Can you work these out from the model? Positions are in its coordinate system, mm. A direction names the side the tool comes from. Coordinates: 2 decimals unless noted, no trailing zeros. Order: outer loops, then holes, each group sorted by start corner. A loop starts at its lowest first (then second) coordinate and runs counter-clockwise, first axis right, second up.
```python
from build123d import *

# Parameters (mm, degrees)
SKETCH1_R      = 2.15
EXTRUDE1_DEPTH = 3


with BuildPart() as part:
    # Sketch1 → Extrude1 (new body)
    with BuildSketch(Plane.XY):
        Polygon((52.497048214, 165), (-27.502951786, 165), (-27.502951786, 115), (-7.502951786, 115), (-7.502951786, 125), (12.497048214, 145), (52.497048214, 145), align=None)
        with Locations((2.497048214, 155)):
            Circle(SKETCH1_R, mode=Mode.SUBTRACT)
        with Locations((42.497048214, 155)):
            Circle(SKETCH1_R, mode=Mode.SUBTRACT)
        with Locations((-17.502951786, 125)):
            Circle(SKETCH1_R, mode=Mode.SUBTRACT)
        with Locations((-17.502951786, 155)):
            Circle(SKETCH1_R, mode=Mode.SUBTRACT)
    extrude(amount=EXTRUDE1_DEPTH)


solid = part.part
```
1. Imagine slicing it at D-D on x = -3.5. Please give me the cut outline in (y, z), then the cut area to 3 significant figures.
Completed:
outline: (129, 0) - (165, 0) - (165, 3) - (129, 3) - close
area: 108 mm2
2. Imagine slicing it at B-B on z = 1.6. Please give me the cut outline in (x, y).
Completed:
outline: (-27.5, 115) - (-7.5, 115) - (-7.5, 125) - (12.5, 145) - (52.5, 145) - (52.5, 165) - (-27.5, 165) - close; hole circle Ø4.3 at (-17.5, 125); hole circle Ø4.3 at (-17.5, 155); hole circle Ø4.3 at (2.5, 155); hole circle Ø4.3 at (42.5, 155)
3. Thinking about a two-plate mould opening in Y: for faces 3 (the cylindrical face through (43.5, 153.1, 1.5)), 4 (the flat face through (3, 146, 0)), 5 (the flat face through (-18, 115, 1)), which applies, pulls with the +Y half, pulls with the -Y half, needs draft (parallel to the pull), parting line crosses it, or undercut?
Completed:
face 3: undercut
face 4: needs draft
face 5: pulls with the -Y half
4. Imagine slicing it at A-A on y = 155. Please give me the cut outline in (x, z), then the cut area to 3 significant figures.
Completed:
outline: (-27.5, 0) - (-19.65, 0) - (-19.65, 3) - (-27.5, 3) - close; (-15.35, 0) - (0.35, 0) - (0.35, 3) - (-15.35, 3) - close; (4.65, 0) - (40.35, 0) - (40.35, 3) - (4.65, 3) - close; (44.65, 0) - (52.5, 0) - (52.5, 3) - (44.65, 3) - close
area: 201 mm2
5. On a 3-axis mill with a long thin cutter (end or side, diameter ignored), from which of +Z, -Z, +X, -X, +Y, -Y can I reach the whole of each face in a straight line? I mean faces 1 (the cylindrical face through (2.03, 152.9, 1.48)), 2 (the flat face through (-7.503, 120, 1)). Say none if no direction works.
Completed:
face 1: +Z, -Z
face 2: +Z, -Z, +X, -Y
6. Imagine slicing it at C-C on x = 33.5. Please give me the cut outline in (y, z).
Completed:
outline: (145, 0) - (165, 0) - (165, 3) - (145, 3) - close
7. Please list where these lines run through material, in increasing order: probe 1 along Y at (x, z) = (42.5, 0.75); probe 2 along X at (y, z) = (155, 1.7); probe 3 along X at (y, z) = (153.5, 2.05).
Completed:
probe 1: y = 145 to 152.85, 157.15 to 165
probe 2: x = -27.5 to -19.65, -15.35 to 0.35, 4.65 to 40.35, 44.65 to 52.5
probe 3: x = -27.5 to -19.04, -15.96 to 0.96, 4.04 to 40.96, 44.04 to 52.5
8. I'm going to push flat-ended pins straight in: pin 1 (1.5 mm diameter, centred on y = 117.5, z = 1.5, fed in from +X); pin 2 (1 mm diameter, centred on x = -1, z = 2, fed in from -Y); pin 3 (0.9 mm diameter, centred on x = 38.5, z = 2, fed in from -Y); pin 4 (2.5 mm diameter, centred on x = -17.5, y = 125, fed in from -Z). Where does each tip first touch, or does it pass through?
Completed:
pin 1: stops at x = -7.5
pin 2: stops at y = 131
pin 3: stops at y = 145
pin 4: passes through
